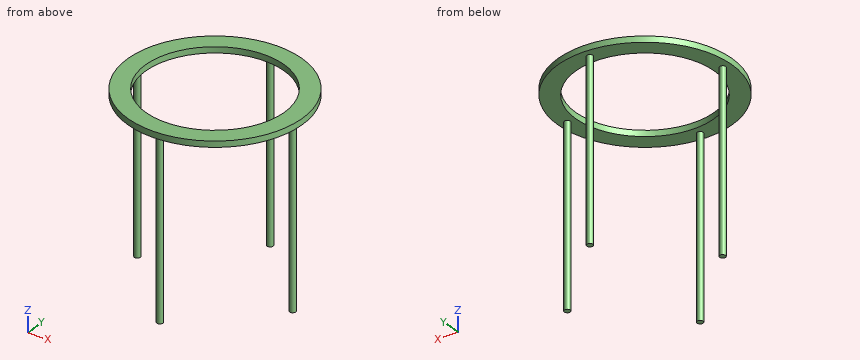
```python
from build123d import *

# Parameters (mm, degrees)
SKETCH2_R           = 146.421356237
SKETCH2_R_2         = 116.421356237
BOSS_EXTRUDE1_DEPTH = 10
SKETCH7_R           = 5
BOSS_EXTRUDE3_DEPTH = 300


with BuildPart() as part:
    # Sketch2 → Boss-Extrude1 (new body)
    with BuildSketch(Plane.XY):
        Circle(SKETCH2_R)
        Circle(SKETCH2_R_2, mode=Mode.SUBTRACT)
    extrude(amount=BOSS_EXTRUDE1_DEPTH)

    # Sketch7 → Boss-Extrude3 (add)
    with BuildSketch(Plane(origin=(0, 0, 0), x_dir=(-1, 0, 0), z_dir=(0, 0, -1))):
        with Locations((-131.421356237, 0)):
            Circle(SKETCH7_R)
        with Locations((0, 131.421356237)):
            Circle(SKETCH7_R)
        with Locations((131.421356237, 0)):
            Circle(SKETCH7_R)
        with Locations((0, -131.421356237)):
            Circle(SKETCH7_R)
    extrude(amount=BOSS_EXTRUDE3_DEPTH)


solid = part.part
```
Read the model definition and answer for the solid it produces. Units are mm, in the model's axes. Coordinates: 2 decimals unless noted, no trailing zeros. Loops run counter-clockwise (first coordinate to the right, second up) from the corner with the lowest first, then second, coordinate; pieces in that order, holes last.
(1) Consider line 1 along Y through (x, z) = (0, 8.25); line 2 along X through (y, z) = (-130.5, -152); line 3 along Z through (x, y) = (120, 29). Determine where each line is inside the solid, lowest interval first.
Solution:
line 1: y = -146.42 to -116.42, 116.42 to 146.42
line 2: x = -4.91 to 4.91
line 3: z = 0 to 10
(2) The part is cut by section C-C (z = -32). Determine the outline of the cut face in (x, y), and give its area (3 significant figures).
Solution:
outline: circle Ø10 at (-131.42, 0); circle Ø10 at (0, -131.42); circle Ø10 at (0, 131.42); circle Ø10 at (131.42, 0)
area: 314 mm2
(3) The part is cut by section D-D (x = 62). Determine the outline of the cut face in (y, z).
Solution:
outline: (-132.65, 0) - (-98.54, 0) - (-98.54, 10) - (-132.65, 10) - close; (98.54, 0) - (132.65, 0) - (132.65, 10) - (98.54, 10) - close
(4) The part is cut by section A-A (y = 0). Determine the outline of the cut face in (x, z), and give its area (3 significant figures).
Solution:
outline: (-146.42, 0) - (-136.42, 0) - (-136.42, -300) - (-126.42, -300) - (-126.42, 0) - (-116.42, 0) - (-116.42, 10) - (-146.42, 10) - close; (116.42, 0) - (126.42, 0) - (126.42, -300) - (136.42, -300) - (136.42, 0) - (146.42, 0) - (146.42, 10) - (116.42, 10) - close
area: 6,600 mm2
